Model file for the job. Use its own axes, mm. A direction names the side the tool comes from. Coordinates: 2 decimals unless noted, no trailing zeros. Write each loop counter-clockwise with the first axis right and the second up, starting at its lowest first coordinate (ties: lowest second). Pieces come first, ordered by that corner, then holes. Notation, with made-up numbers: (73.25, 40.25) - (108.25, 40.25) arc R22 ccw to (108.25, 62.25) - close; hole circle Ø3 at (87, -16). An arc over 180 degrees is marked (long way). Put each result on its own line as item: value. Start each with the question number.
1. Saw through at A-A, the plane z = -41. Write the cut outline in (x, y).
2. Pull direction X, two halves, no side cores. Call faces 1 (the face through (-30.92, 2.41, 109.93)), 2 (the face through (-1, 0, 31)), 3 (the face through (45.414, 2.415, 71.765)): released by +X, released by -X, zero draft, split by the parting line, or undercut.
3. Saw through at B-B, the plane x = -35. Write the cut outline in (y, z), plus the area to 3 significant figures.
4. Saw through at C-C, the plane z = 65. Write the cut outline in (x, y).
5. Drill centre lines: L1, parallel to X at y = 2.75, z = -36.5; L2, parallel to Z at x = -84, y = 2.8; L3, parallel to Y at x = -75, z = -148. Where is each one in solid material? Low to high. Write a range as from..to.
6. Which spindle directions (+Z, -Z, +X, -X, +Y, -Y) get a long thin tool onto all of the face, cutting with end or side? Do faces 4 (the face through (-1, 4.762, 31)), 5 (the face through (-45.414, 2.415, 108.235)). Say none if no direction does.
```python
from build123d import *

# Parameters (mm, degrees)
SKETCH1_W                            = 200
SKETCH1_H                            = 300
BOSS_EXTRUDE1_DEPTH                  = 4.7625
F_1_4_20_TAPPED_HOLE1_D              = 5.1054
M4X0_7_TAPPED_HOLE1_D                = 3.3
M5_CLEARANCE_HOLE1_D                 = 5.3
SKETCH9_W                            = 63
SKETCH9_H                            = 81
SKETCH9_W_2                          = 29.5
SKETCH9_H_2                          = 79
SKETCH9_H_3                          = 37
SKETCH9_H_4                          = 30
CUT_EXTRUDE1_DEPTH                   = 181.340459704
TAP_DRILL_FOR_M3X0_5_TAP1_AT_2_COUNT = 2
TAP_DRILL_FOR_M3X0_5_TAP1_AT_2_PITCH = 150
TAP_DRILL_FOR_M3X0_5_TAP2_AT_2_COUNT = 2
TAP_DRILL_FOR_M3X0_5_TAP2_AT_2_PITCH = 275
TAP_DRILL_FOR_M3X0_5_TAP2_AT_3_COUNT = 2
TAP_DRILL_FOR_M3X0_5_TAP2_AT_3_PITCH = 137.5
FILLET1_R                            = 3
FILLET2_R                            = 1


with BuildPart() as part:
    # Sketch1 → Boss-Extrude1 (new body)
    with BuildSketch(Plane(origin=(0, 0, 0), x_dir=(1, 0, 0), z_dir=(0, 1, 0))):
        Rectangle(SKETCH1_W, SKETCH1_H)
    extrude(amount=BOSS_EXTRUDE1_DEPTH)

    # 1/4-20 Tapped Hole1 (through all)
    with Locations(Plane(origin=(0, 4.7625, 0), x_dir=(1, 0, 0), z_dir=(0, 1, 0))):
        with Locations((-87.3, -84.6), (-87.3, -135.4), (87.3, -135.4), (87.3, -84.6)):
            Hole(F_1_4_20_TAPPED_HOLE1_D / 2)

    # M4x0.7 Tapped Hole1 (through all)
    with Locations(Plane(origin=(0, 4.7625, 0), x_dir=(1, 0, 0), z_dir=(0, 1, 0))):
        with Locations((-14.75, 11), (14.75, 11), (14.75, 100), (-14.75, 100)):
            Hole(M4X0_7_TAPPED_HOLE1_D / 2)

    # M5 Clearance Hole1 (through all)
    with Locations(Plane(origin=(0, 4.7625, 0), x_dir=(1, 0, 0), z_dir=(0, 1, 0))):
        with Locations((-60, 10), (-60, -140), (60, -140), (60, 10)):
            Hole(M5_CLEARANCE_HOLE1_D / 2)

    # Sketch9 → Cut-Extrude1 (cut, through all)
    with BuildSketch(Plane(origin=(0, 4.7625, 0), x_dir=(1, 0, 0), z_dir=(0, 1, 0))):
        Polygon((-80, -54.472135955), (-80, -125.527864045), (-8.94427191, -90), align=None)
        Polygon((-71.05572809, -50), (71.05572809, -50), (0, -85.527864045), align=None)
        Polygon((80, -54.472135955), (8.94427191, -90), (80, -125.527864045), align=None)
        Polygon((-71.05572809, -130), (0, -94.472135955), (71.05572809, -130), align=None)
        with Locations((-56.5, 101.5)):
            Rectangle(SKETCH9_W, SKETCH9_H)
        with Locations((56.5, 101.5)):
            Rectangle(SKETCH9_W, SKETCH9_H)
        with Locations((0, 55.5)):
            Rectangle(SKETCH9_W_2, SKETCH9_H_2)
        with Locations((0, 123.5)):
            Rectangle(SKETCH9_W_2, SKETCH9_H_3)
        with Locations((0, -11.5)):
            Rectangle(SKETCH9_W_2, SKETCH9_H_3)
        with Locations((-56.5, 36)):
            Rectangle(SKETCH9_W, SKETCH9_H_4)
        with Locations((-56.5, -15)):
            Rectangle(SKETCH9_W, SKETCH9_H_4)
        with Locations((56.5, -15)):
            Rectangle(SKETCH9_W, SKETCH9_H_4)
        with Locations((56.5, 36)):
            Rectangle(SKETCH9_W, SKETCH9_H_4)
    extrude(amount=-CUT_EXTRUDE1_DEPTH, mode=Mode.SUBTRACT)

    # Sketch12 → Tap Drill for M3x0.5 Tap1 (revolve, cut)
    with BuildSketch(Plane(origin=(-75, 2.38125, 150), x_dir=(0, -1, 0), z_dir=(1, 0, 0))):
        Polygon((0, 0), (0, 5.511075774), (1.25, 4.76), (1.25, 0), align=None)
    tap_drill_for_m3x0_5_tap1 = revolve(axis=Axis((-75, 2.38125, 156.35), (0, 0, -1)), mode=Mode.SUBTRACT)

    # Tap Drill for M3x0.5 Tap1 at 2: Tap Drill for M3x0.5 Tap1 ×2
    with Locations(*[(i * TAP_DRILL_FOR_M3X0_5_TAP1_AT_2_PITCH, 0, 0) for i in range(1, TAP_DRILL_FOR_M3X0_5_TAP1_AT_2_COUNT)]):
        add(tap_drill_for_m3x0_5_tap1, mode=Mode.SUBTRACT)

    # Mirror1: Tap Drill for M3x0.5 Tap1 across plane
    add(tap_drill_for_m3x0_5_tap1.mirror(Plane.XY), mode=Mode.SUBTRACT)

    # Mirror1 copy 1 sketch → Mirror1 copy 1 (revolve, cut)
    with BuildSketch(Plane(origin=(75, 2.38125, -150), x_dir=(0, -1, 0), z_dir=(1, 0, 0))):
        Polygon((0, 0), (0, -5.511075774), (1.25, -4.76), (1.25, 0), align=None)
    revolve(axis=Axis((75, 2.38125, -156.35), (0, 0, -1)), mode=Mode.SUBTRACT)

    # Sketch15 → Tap Drill for M3x0.5 Tap2 (revolve, cut)
    with BuildSketch(Plane(origin=(-100, 2.38125, -137.5), x_dir=(0, 0, 1), z_dir=(0, 1, 0))):
        Polygon((0, 0), (0, 5.511075774), (1.25, 4.76), (1.25, 0), align=None)
    tap_drill_for_m3x0_5_tap2 = revolve(axis=Axis((-106.35, 2.38125, -137.5), (1, 0, 0)), mode=Mode.SUBTRACT)

    # Tap Drill for M3x0.5 Tap2 at 2: Tap Drill for M3x0.5 Tap2 ×2
    with Locations(*[(0, 0, i * TAP_DRILL_FOR_M3X0_5_TAP2_AT_2_PITCH) for i in range(1, TAP_DRILL_FOR_M3X0_5_TAP2_AT_2_COUNT)]):
        add(tap_drill_for_m3x0_5_tap2, mode=Mode.SUBTRACT)

    # Tap Drill for M3x0.5 Tap2 at 3: Tap Drill for M3x0.5 Tap2 ×2
    with Locations(*[(0, 0, i * TAP_DRILL_FOR_M3X0_5_TAP2_AT_3_PITCH) for i in range(1, TAP_DRILL_FOR_M3X0_5_TAP2_AT_3_COUNT)]):
        add(tap_drill_for_m3x0_5_tap2, mode=Mode.SUBTRACT)

    # Mirror2: Tap Drill for M3x0.5 Tap2 across plane
    add(tap_drill_for_m3x0_5_tap2.mirror(Plane(origin=(0, 0, 0), x_dir=(0, 0, 1), z_dir=(1, 0, 0))), mode=Mode.SUBTRACT)

    # Mirror2 copy 1 sketch → Mirror2 copy 1 (revolve, cut)
    with BuildSketch(Plane(origin=(100, 2.38125, 137.5), x_dir=(0, 0, 1), z_dir=(0, 1, 0))):
        Polygon((0, 0), (0, -5.511075774), (1.25, -4.76), (1.25, 0), align=None)
    revolve(axis=Axis((106.35, 2.38125, 137.5), (1, 0, 0)), mode=Mode.SUBTRACT)

    # Mirror2 copy 2 sketch → Mirror2 copy 2 (revolve, cut)
    with BuildSketch(Plane(origin=(100, 2.38125, 0), x_dir=(0, 0, 1), z_dir=(0, 1, 0))):
        Polygon((0, 0), (0, -5.511075774), (1.25, -4.76), (1.25, 0), align=None)
    revolve(axis=Axis((106.35, 2.38125, 0), (1, 0, 0)), mode=Mode.SUBTRACT)

    # Fillet1
    fillet1_edges = [part.edges().sort_by_distance(p)[0] for p in [
        (14.75, 2.38125, -95),
        (14.75, 2.38125, -16),
        (-14.75, 2.38125, -16),
        (-14.75, 2.38125, -95),
        (25, 2.38125, 30),
        (25, 2.38125, 0),
        (88, 2.38125, 0),
        (88, 2.38125, 30),
        (88, 2.38125, -142),
        (88, 2.38125, -61),
        (25, 2.38125, -61),
        (25, 2.38125, -142),
        (-88, 2.38125, 30),
        (-88, 2.38125, 0),
        (-25, 2.38125, 0),
        (-25, 2.38125, 30),
        (71.05572809, 2.38125, 130),
        (-71.05572809, 2.38125, 130),
        (0, 2.38125, 94.472135955),
        (80, 2.38125, 54.472135955),
        (80, 2.38125, 125.527864045),
        (8.94427191, 2.38125, 90),
        (-80, 2.38125, 54.472135955),
        (-8.94427191, 2.38125, 90),
        (-80, 2.38125, 125.527864045),
        (0, 2.38125, 85.527864045),
        (-71.05572809, 2.38125, 50),
        (71.05572809, 2.38125, 50),
        (25, 2.38125, -21),
        (25, 2.38125, -51),
        (88, 2.38125, -51),
        (88, 2.38125, -21),
        (-25, 2.38125, -51),
        (-25, 2.38125, -21),
        (-88, 2.38125, -21),
        (-88, 2.38125, -51),
        (14.75, 2.38125, -7),
        (14.75, 2.38125, 30),
        (-14.75, 2.38125, 30),
        (-14.75, 2.38125, -7),
        (14.75, 2.38125, -142),
        (14.75, 2.38125, -105),
        (-14.75, 2.38125, -105),
        (-14.75, 2.38125, -142),
        (-25, 2.38125, -142),
        (-25, 2.38125, -61),
        (-88, 2.38125, -61),
        (-88, 2.38125, -142),
    ]]
    fillet(fillet1_edges, radius=FILLET1_R)

    # Fillet2
    fillet2_edges = [part.edges().sort_by_distance(p)[0] for p in [
        (100, 2.38125, 150),
        (-100, 2.38125, 150),
        (-100, 2.38125, -150),
        (100, 2.38125, -150),
    ]]
    fillet(fillet2_edges, radius=FILLET2_R)


solid = part.part
```
Final values:
1. outline: (-100, 0) - (-88, 0) - (-88, 4.76) - (-100, 4.76) - close; (-25, 0) - (-14.75, 0) - (-14.75, 4.76) - (-25, 4.76) - close; (14.75, 0) - (25, 0) - (25, 4.76) - (14.75, 4.76) - close; (88, 0) - (100, 0) - (100, 4.76) - (88, 4.76) - close
2. face 1: undercut
2. face 2: zero draft
2. face 3: undercut
3. outline: (0, -150) - (4.76, -150) - (4.76, -142) - (0, -142) - close; (0, -61) - (4.76, -61) - (4.76, -51) - (0, -51) - close; (0, -21) - (4.76, -21) - (4.76, 0) - (0, 0) - close; (0, 30) - (4.76, 30) - (4.76, 50) - (0, 50) - close; (0, 68.03) - (4.76, 68.03) - (4.76, 76.97) - (0, 76.97) - close; (0, 103.03) - (4.76, 103.03) - (4.76, 111.97) - (0, 111.97) - close; (0, 130) - (4.76, 130) - (4.76, 150) - (0, 150) - close
3. area: 461 mm²
4. outline: (-100, 0) - (-80, 0) - (-80, 4.76) - (-100, 4.76) - close; (-58.94, 0) - (-41.06, 0) - (-41.06, 4.76) - (-58.94, 4.76) - close; (41.06, 0) - (58.94, 0) - (58.94, 4.76) - (41.06, 4.76) - close; (80, 0) - (100, 0) - (100, 4.76) - (80, 4.76) - close
5. L1: x = -100..-88, -25..-14.75, 14.75..25, 88..100
5. L2: z = -150..-142, -61..-51, -21..0, 30..150
5. L3: y = 0..1.13, 3.63..4.76
6. face 4: +Z, -Z, +X, -X, +Y
6. face 5: +Y, -Y
